Check sheet for the modelled part. Datum: model origin and axes. Units: mm. A direction names the side the tool comes from. Round coordinates to 2 decimals unless told otherwise and drop trailing zeros. Order: outer loops, then holes, each group sorted by start corner. A loop starts at its lowest first (then second) coordinate and runs counter-clockwise, first axis right, second up. Notation, with made-up numbers: (11.25, 32) -> (25.25, 32) arc R12 ccw to (25.25, 39) -> close; hole circle Ø6 at (74.5, 2). An arc over 180 degrees is marked (long way). Answer in a Markdown table with one row per item. Add a question column.
1. Access from +Z, -Z, +X, -X, +Y, -Y to the whole of each face (thin tool, end or side, straight path). Record for faces 4 (the flat face through (25.4, 238, -13)), 5 (the flat face through (13, 238, -24.13)).
2. Sectioned sample at A-A, the plane z = -11. Record the boundary of the cut face in (x, y).
3. Sectioned sample at B-B, the plane y = 273.5. Record the boundary of the cut face in (x, z), then the cut area to 3 significant figures.
4. Depth check by flat-ended pin: P1, Ø2, axis at x = 3.5, z = -22, coming from the -Y side; P2, Ø6, axis at x = 2.5, z = -3, coming from the -Y side; P3, Ø4.5, axis at x = 12.72, y = 18.42, coming from the -Z side. Enter the tip coordinate at first touch or a pass-through.
5. Material ranges on L1, parallel to Y at x = 12.7, z = -0.5; L2, parallel to X at y = 223.6, z = -0.75; L3, parallel to X at y = 358.5, z = -13, recorded low to high. Write a range as from..to.
6. Draft check along Z on faces 1 (the flat face through (1.27, 238, -13)), 2 (the flat face through (13, 238, 0)), 3 (the flat face through (12, 482.6, -1)). Enter one of: +Z half, -Z half, draft (parallel to the pull), parting line (faces both ways), or undercut.
```python
from build123d import *

# Parameters (mm, degrees)
SKETCH1_W           = 25.4
SKETCH1_H           = 25.4
BOSS_EXTRUDE1_DEPTH = 482.6
SKETCH3_R           = 2.54
CUT_EXTRUDE1_DEPTH  = 2.54
SKETCH4_R           = 2.54
CUT_EXTRUDE2_DEPTH  = 2.54
SKETCH5_R           = 2.54
CUT_EXTRUDE3_DEPTH  = 2.54
SKETCH6_R           = 3.556
CUT_EXTRUDE4_DEPTH  = 2.54
SKETCH7_R           = 3.556
CUT_EXTRUDE5_DEPTH  = 2.54


with BuildPart() as part:
    # Sketch1 → Boss-Extrude1 (new body)
    with BuildSketch(Plane(origin=(0, 0, 0), x_dir=(1, 0, 0), z_dir=(0, 1, 0))):
        with Locations((12.7, 12.7)):
            Rectangle(SKETCH1_W, SKETCH1_H)
        Polygon((1.27, 12.361459156), (1.27, 24.13), (12.7, 24.13), (24.13, 24.13), (24.13, 12.7), (24.13, 1.27), (12.7, 1.27), (1.27, 1.27), align=None, mode=Mode.SUBTRACT)
    extrude(amount=BOSS_EXTRUDE1_DEPTH)

    # Sketch3 → Cut-Extrude1 (cut)
    with BuildSketch(Plane(origin=(0, 0, -25.4), x_dir=(-1, 0, 0), z_dir=(0, 0, -1))):
        with Locations((-12.762028981, 449.168015032)):
            Circle(SKETCH3_R)
    extrude(amount=-CUT_EXTRUDE1_DEPTH, mode=Mode.SUBTRACT)

    # Sketch4 → Cut-Extrude2 (cut)
    with BuildSketch(Plane(origin=(0, 0, -25.4), x_dir=(-1, 0, 0), z_dir=(0, 0, -1))):
        with Locations((-12.70057371, 321.200750094)):
            Circle(SKETCH4_R)
    extrude(amount=-CUT_EXTRUDE2_DEPTH, mode=Mode.SUBTRACT)

    # Sketch5 → Cut-Extrude3 (cut)
    with BuildSketch(Plane(origin=(0, 0, -25.4), x_dir=(-1, 0, 0), z_dir=(0, 0, -1))):
        with Locations((-12.715968996, 18.41791766)):
            Circle(SKETCH5_R)
    extrude(amount=-CUT_EXTRUDE3_DEPTH, mode=Mode.SUBTRACT)

    # Sketch6 → Cut-Extrude4 (cut)
    with BuildSketch(Plane.XY):
        with Locations((12.7, 63.552)):
            Circle(SKETCH6_R)
    extrude(amount=-CUT_EXTRUDE4_DEPTH, mode=Mode.SUBTRACT)

    # Sketch7 → Cut-Extrude5 (cut)
    with BuildSketch(Plane.XY):
        with Locations((12.7, 223.6)):
            Circle(SKETCH7_R)
        with Locations((12.7, 319.6)):
            Circle(SKETCH7_R)
    extrude(amount=-CUT_EXTRUDE5_DEPTH, mode=Mode.SUBTRACT)


solid = part.part
```
Answer key:
| question | item | result |
|---|---|---|
| 1 | face 4 | +Z, -Z, +X, +Y, -Y |
| 1 | face 5 | +Y, -Y |
| 2 | outline | (0, 0) -> (1.27, 0) -> (1.27, 482.6) -> (0, 482.6) -> close; (24.13, 0) -> (25.4, 0) -> (25.4, 482.6) -> (24.13, 482.6) -> close |
| 3 | outline | (0, -25.4) -> (25.4, -25.4) -> (25.4, 0) -> (0, 0) -> close; hole (1.27, -24.13) -> (24.13, -24.13) -> (24.13, -1.27) -> (1.27, -1.27) -> close |
| 3 | area | 123 mm² |
| 4 | P1 | passes through |
| 4 | P2 | stops at y = 0 |
| 4 | P3 | stops at z = -1.27 |
| 5 | L1 | y = 0..60, 67.11..220.04, 227.16..316.04, 323.16..482.6 |
| 5 | L2 | x = 0..9.14, 16.26..25.4 |
| 5 | L3 | x = 0..1.27, 24.13..25.4 |
| 6 | face 1 | undercut |
| 6 | face 2 | +Z half |
| 6 | face 3 | draft |
